Part model, mm, in its own coordinate system. Give positions to 0.01 mm unless a question says otherwise; leave off trailing zeros. Write each loop counter-clockwise with the first axis right and the second up, starting at its lowest first coordinate (ties: lowest second). Pieces come first, ordered by that corner, then holes.
```python
from build123d import *


with BuildPart() as f1:
    # F0 (on Front) → F1 (revolve)
    with BuildSketch(Plane.XZ):
        with BuildLine():
            Line((0, 21.6693256305), (0, 0))
            Line((0, 0), (150, 0))
            Line((150, 0), (150, 17.5))
            Line((150, 17.5), (110, 17.5))
            Line((110, 17.5), (110, 30))
            Line((110, 30), (90, 30))
            Line((90, 30), (90, 17.5))
            Line((90, 17.5), (77.4651691318, 6.678994745))
            add(Edge.make_bspline(
                [(72.9966231084, 15.6097216852), (75.1787620527, 12.4225102506), (76.3219655922, 9.5507524978), (77.4651691318, 6.678994745)],
                knots=[0.7288272916, 0.7288272916, 0.7288272916, 0.7288272916, 1, 1, 1, 1], degree=3))
            add(Edge.make_bspline(
                [(71.5628042817, 17.5517760217), (72.0873115849, 16.8902851499), (72.562524827, 16.2437615157), (72.9966231084, 15.6097216852)],
                knots=[0.6748822361, 0.6748822361, 0.6748822361, 0.6748822361, 0.7288272916, 0.7288272916, 0.7288272916, 0.7288272916], degree=3))
            add(Edge.make_bspline(
                [(64.663942956, 24.3176637406), (66.9289575988, 22.7303573773), (69.5933719963, 20.0355574133), (71.5628042817, 17.5517760217)],
                knots=[0.4723280801, 0.4723280801, 0.4723280801, 0.4723280801, 0.6748822361, 0.6748822361, 0.6748822361, 0.6748822361], degree=3))
            Line((64.663942956, 24.3176637406), (61.000674963, 25.6286989897))
            add(Edge.make_bspline(
                [(59.830175783, 20.9419401689), (59.6901790229, 23.437797919), (59.945740487, 25.2370869651), (61.000674963, 25.6286989897)],
                knots=[0.167170672, 0.167170672, 0.167170672, 0.167170672, 0.3378307298, 0.3378307298, 0.3378307298, 0.3378307298], degree=3))
            add(Edge.make_bspline(
                [(61.000674963, 12.270710431), (60.4839925374, 15.3839120928), (59.9673101118, 18.4971137545), (59.830175783, 20.9419401689)],
                knots=[0, 0, 0, 0, 0.167170672, 0.167170672, 0.167170672, 0.167170672], degree=3))
            Line((61.000674963, 12.270710431), (57.1930049726, 7.9697840538))
            Line((57.1930049726, 7.9697840538), (56.4116936669, 12.8312731816))
            Line((56.4116936669, 12.8312731816), (52.9237501323, 12.270710431))
            Line((52.9237501323, 12.270710431), (50.127889961, 29.6671614051))
            Line((50.127889961, 29.6671614051), (46.0894331336, 12.270710431))
            Line((46.0894331336, 12.270710431), (43.2935729623, 29.6671614051))
            Line((43.2935729623, 29.6671614051), (39.5657643676, 12.270710431))
            Line((39.5657643676, 12.270710431), (36.7699041963, 29.6671614051))
            Line((36.7699041963, 29.6671614051), (33.6633957922, 12.270710431))
            Line((33.6633957922, 12.270710431), (30.8675356209, 29.6671614051))
            Line((30.8675356209, 29.6671614051), (27.7610272169, 12.270710431))
            Line((27.7610272169, 12.270710431), (24.0332167596, 12.270710431))
            Line((24.0332167596, 12.270710431), (21.8586623669, 8.232248947))
            Line((21.8586623669, 8.232248947), (19.0628003329, 12.270710431))
            add(Edge.make_bspline(
                [(18.5265220099, 15.8898699265), (18.7097725422, 14.6979257427), (18.8862864375, 13.4843180868), (19.0628003329, 12.270710431)],
                knots=[0.924417358, 0.924417358, 0.924417358, 0.924417358, 1, 1, 1, 1], degree=3))
            add(Edge.make_bspline(
                [(17.8406653269, 19.9722953613), (18.0859294682, 18.6650141612), (18.3108896528, 17.2924401159), (18.5265220099, 15.8898699265)],
                knots=[0.8354786627, 0.8354786627, 0.8354786627, 0.8354786627, 0.924417358, 0.924417358, 0.924417358, 0.924417358], degree=3))
            Line((17.8406653269, 19.9722953613), (17.1299511809, 23.282187563))
            add(Edge.make_bspline(
                [(15.8701302608, 27.1433569712), (16.3522663189, 26.0563077049), (16.7649165996, 24.7458081918), (17.1299511809, 23.282187563)],
                knots=[0.6444204964, 0.6444204964, 0.6444204964, 0.6444204964, 0.7563362266, 0.7563362266, 0.7563362266, 0.7563362266], degree=3))
            Line((15.8701302608, 27.1433569712), (14.8938185182, 28.8829312407))
            add(Edge.make_bspline(
                [(13.1604354829, 30.2884634584), (13.8127999128, 30.0597529266), (14.3855904242, 29.5751510115), (14.8938185182, 28.8829312407)],
                knots=[0.4766859999, 0.4766859999, 0.4766859999, 0.4766859999, 0.575408405, 0.575408405, 0.575408405, 0.575408405], degree=3))
            add(Edge.make_bspline(
                [(12.04068262, 30.443642999), (12.4352655238, 30.4605151191), (12.8093725631, 30.4115415776), (13.1604354829, 30.2884634584)],
                knots=[0.4235595966, 0.4235595966, 0.4235595966, 0.4235595966, 0.4766859999, 0.4766859999, 0.4766859999, 0.4766859999], degree=3))
            add(Edge.make_bspline(
                [(9.7332416868, 29.7643078399), (10.558441204, 30.1710049421), (11.3325366462, 30.4133631166), (12.04068262, 30.443642999)],
                knots=[0.3282152515, 0.3282152515, 0.3282152515, 0.3282152515, 0.4235595966, 0.4235595966, 0.4235595966, 0.4235595966], degree=3))
            add(Edge.make_bspline(
                [(9.0672849858, 29.4075766104), (9.2926696096, 29.5374176038), (9.5147470344, 29.6566234071), (9.7332416868, 29.7643078399)],
                knots=[0.3029701695, 0.3029701695, 0.3029701695, 0.3029701695, 0.3282152515, 0.3282152515, 0.3282152515, 0.3282152515], degree=3))
            add(Edge.make_bspline(
                [(6.5741276375, 27.678059166), (7.438193805, 28.3607294899), (8.2732626939, 28.9501512486), (9.0672849858, 29.4075766104)],
                knots=[0.2140326121, 0.2140326121, 0.2140326121, 0.2140326121, 0.3029701695, 0.3029701695, 0.3029701695, 0.3029701695], degree=3))
            add(Edge.make_bspline(
                [(2.2138374421, 23.8062424173), (3.7090372266, 25.2311697916), (5.1793602452, 26.5760992199), (6.5741276375, 27.678059166)],
                knots=[0.0704704525, 0.0704704525, 0.0704704525, 0.0704704525, 0.2140326121, 0.2140326121, 0.2140326121, 0.2140326121], degree=3))
            add(Edge.make_bspline(
                [(0, 21.6693256305), (0.7399438662, 22.3880565014), (1.4798877324, 23.1067873722), (2.2138374421, 23.8062424173)],
                knots=[0, 0, 0, 0, 0.0704704525, 0.0704704525, 0.0704704525, 0.0704704525], degree=3))
        make_face()
        with BuildLine():
            Line((1.2346615549, 25.5908425897), (0, 21.6693256305))
            add(Edge.make_bspline(
                [(0, 21.6693256305), (0.7399438662, 22.3880565014), (1.4798877324, 23.1067873722), (2.2138374421, 23.8062424173)],
                knots=[0, 0, 0, 0, 0.0704704525, 0.0704704525, 0.0704704525, 0.0704704525], degree=3))
            Line((2.2138374421, 23.8062424173), (1.2346615549, 25.5908425897))
        make_face()
        with BuildLine():
            Line((6.5741276375, 33.3432426597), (6.5741276375, 27.678059166))
            add(Edge.make_bspline(
                [(6.5741276375, 27.678059166), (7.438193805, 28.3607294899), (8.2732626939, 28.9501512486), (9.0672849858, 29.4075766104)],
                knots=[0.2140326121, 0.2140326121, 0.2140326121, 0.2140326121, 0.3029701695, 0.3029701695, 0.3029701695, 0.3029701695], degree=3))
            Line((9.0672849858, 29.4075766104), (6.5741276375, 33.3432426597))
        make_face()
        with BuildLine():
            Line((10.5205139602, 34.5443420431), (9.7332416868, 29.7643078399))
            add(Edge.make_bspline(
                [(9.7332416868, 29.7643078399), (10.558441204, 30.1710049421), (11.3325366462, 30.4133631166), (12.04068262, 30.443642999)],
                knots=[0.3282152515, 0.3282152515, 0.3282152515, 0.3282152515, 0.4235595966, 0.4235595966, 0.4235595966, 0.4235595966], degree=3))
            Line((12.04068262, 30.443642999), (10.5205139602, 34.5443420431))
        make_face()
        with BuildLine():
            Line((16.2498224527, 34.0652950108), (13.1604354829, 30.2884634584))
            add(Edge.make_bspline(
                [(13.1604354829, 30.2884634584), (13.8127999128, 30.0597529266), (14.3855904242, 29.5751510115), (14.8938185182, 28.8829312407)],
                knots=[0.4766859999, 0.4766859999, 0.4766859999, 0.4766859999, 0.575408405, 0.575408405, 0.575408405, 0.575408405], degree=3))
            Line((14.8938185182, 28.8829312407), (16.2498224527, 34.0652950108))
        make_face()
        with BuildLine():
            add(Edge.make_bspline(
                [(71.5628042817, 17.5517760217), (72.0873115849, 16.8902851499), (72.562524827, 16.2437615157), (72.9966231084, 15.6097216852)],
                knots=[0.6748822361, 0.6748822361, 0.6748822361, 0.6748822361, 0.7288272916, 0.7288272916, 0.7288272916, 0.7288272916], degree=3))
            Line((72.9966231084, 15.6097216852), (78.7995061792, 30.0915367624))
            Line((78.7995061792, 30.0915367624), (71.5628042817, 17.5517760217))
        make_face()
        with BuildLine():
            add(Edge.make_bspline(
                [(14.8938185182, 28.8829312407), (15.2490963671, 28.399033648), (15.5728242636, 27.8136786793), (15.8701302608, 27.1433569712)],
                knots=[0.575408405, 0.575408405, 0.575408405, 0.575408405, 0.6444204964, 0.6444204964, 0.6444204964, 0.6444204964], degree=3))
            Line((14.8938185182, 28.8829312407), (15.8701302608, 27.1433569712))
        make_face()
        with BuildLine():
            Line((20.0848666792, 27.1433569712), (15.8701302608, 27.1433569712))
            add(Edge.make_bspline(
                [(15.8701302608, 27.1433569712), (16.3522663189, 26.0563077049), (16.7649165996, 24.7458081918), (17.1299511809, 23.282187563)],
                knots=[0.6444204964, 0.6444204964, 0.6444204964, 0.6444204964, 0.7563362266, 0.7563362266, 0.7563362266, 0.7563362266], degree=3))
            Line((17.1299511809, 23.282187563), (20.0848666792, 27.1433569712))
        make_face()
        with BuildLine():
            Line((61.000674963, 25.6286989897), (64.663942956, 24.3176637406))
            add(Edge.make_bspline(
                [(61.000674963, 25.6286989897), (61.8320698045, 25.9373287905), (63.1599576823, 25.3716460638), (64.663942956, 24.3176637406)],
                knots=[0.3378307298, 0.3378307298, 0.3378307298, 0.3378307298, 0.4723280801, 0.4723280801, 0.4723280801, 0.4723280801], degree=3))
        make_face()
        with BuildLine():
            add(Edge.make_bspline(
                [(61.000674963, 25.6286989897), (61.8320698045, 25.9373287905), (63.1599576823, 25.3716460638), (64.663942956, 24.3176637406)],
                knots=[0.3378307298, 0.3378307298, 0.3378307298, 0.3378307298, 0.4723280801, 0.4723280801, 0.4723280801, 0.4723280801], degree=3))
            Line((64.663942956, 24.3176637406), (56.147307816, 40.1663766136))
            Line((56.147307816, 40.1663766136), (59.830175783, 20.9419401689))
            add(Edge.make_bspline(
                [(59.830175783, 20.9419401689), (59.6901790229, 23.437797919), (59.945740487, 25.2370869651), (61.000674963, 25.6286989897)],
                knots=[0.167170672, 0.167170672, 0.167170672, 0.167170672, 0.3378307298, 0.3378307298, 0.3378307298, 0.3378307298], degree=3))
        make_face()
        with BuildLine():
            add(Edge.make_bspline(
                [(17.1299511809, 23.282187563), (17.3880893889, 22.2471721816), (17.6224160983, 21.1355845078), (17.8406653269, 19.9722953613)],
                knots=[0.7563362266, 0.7563362266, 0.7563362266, 0.7563362266, 0.8354786627, 0.8354786627, 0.8354786627, 0.8354786627], degree=3))
            Line((17.1299511809, 23.282187563), (17.8406653269, 19.9722953613))
        make_face()
        with BuildLine():
            Line((21.1058293493, 20.6734052822), (17.8406653269, 19.9722953613))
            add(Edge.make_bspline(
                [(17.8406653269, 19.9722953613), (18.0859294682, 18.6650141612), (18.3108896528, 17.2924401159), (18.5265220099, 15.8898699265)],
                knots=[0.8354786627, 0.8354786627, 0.8354786627, 0.8354786627, 0.924417358, 0.924417358, 0.924417358, 0.924417358], degree=3))
            Line((18.5265220099, 15.8898699265), (21.1058293493, 20.6734052822))
        make_face()
    revolve(axis=Axis((75, 0, 0), (1, 0, 0)))

    # F2: F1 across face


with BuildPart() as f1_1:
    add(f1.part)
    add(f1.part.mirror(Plane(origin=(0, 0, 0), x_dir=(0, -1, 0), z_dir=(-1, 0, 0))))


solid = f1_1.part
```
1) Saw through at B-B, the plane x = 120.5. Write the cut outline in (y, z), then the cut area to 3 significant figures.
Answers follow:
outline: circle Ø35 at (0, 0)
area: 962 mm2
2) Saw through at A-A, the plane y = -8.5. Count the separate pieces of the cut face and the enclosed holes in it, then the cut area to 3 significant figures.
Answers follow:
separate pieces: 7
enclosed holes: 0
area: 11,000 mm2
3) Two-plate mould, pull along Z, no slides. Class faces 1 (the face through (64.13, 24.71, -5.49)), 2 (the face through (-6.574, -25, -13)), 3 (the face through (-57.144, -2.485, 7.892)): +Z half, -Z half, draft (parallel to the pull), parting line (faces both ways), or undercut.
Answers follow:
face 1: parting line
face 2: draft
face 3: undercut
4) Wall check: L1, parallel to X at y = 36, z = 2.5; L2, parallel to Y at x = -66, z = 1.5; L3, parallel to Y at x = 115.5, z = -14. Give the ranges that are in metal, low to high.
Answers follow:
L1: x = -58.34 to -56.93, 56.93 to 58.34
L2: y = -23.25 to 23.25
L3: y = -10.5 to 10.5
5) Saw through at C-C, the plane x = -98. Write the cut outline in (y, z).
Answers follow:
outline: circle Ø60 at (0, 0)
6) Pin check, flat tips, straight feed: pin 1 Ø2 at (x, z) = (8.5, 1) entering from -Y; pin 2 Ø1 at (x, z) = (64, 13) entering from -Y; pin 3 Ø10 at (x, z) = (115.5, -26.5) entering from +Y; pin 4 Ø2 at (x, y) = (-108.5, -8) entering from +Z. Stop position of each tip, or through.
Answers follow:
pin 1: stops at y = -31.87
pin 2: stops at y = -23.11
pin 3: passes through
pin 4: stops at z = 29.17
